For this review, take the finished solid that the model builds, in its own axes (mm). A direction names the side the tool comes from. Give positions to 0.01 mm unless a question says otherwise; leave off trailing zeros. Write each loop counter-clockwise with the first axis right and the second up, starting at its lowest first coordinate (ties: lowest second). Pieces come first, ordered by that corner, then holes.
from build123d import *

# Parameters (mm, degrees)
F0_W      = 38.1
F0_H      = 38.1
F1_DEPTH  = 0.79375
F2_W      = 38.1
F2_H      = 38.1
F2_W_2    = 34.8996
F2_H_2    = 34.8996
F3_DEPTH  = 5.08
F4_W      = 1.27
F4_H      = 10.9915577808
F4_H_2    = 10.7192572
F5_DEPTH  = 4.445
F7_W      = 1.27
F7_H      = 6.305353716
F9_DEPTH  = 4.445
F8_W      = 1.27
F8_H      = 7.127109261
F8_H_2    = 15.866300866
F8_W_2    = 9.8573208662
F8_H_3    = 1.27
F10_DEPTH = 4.445
F11_W     = 8.128
F11_H     = 1.27
F12_DEPTH = 4.445


# Not quite as in the source:
# - a feature names something its author has since deleted; it is built from what else it names


with BuildPart() as f1:
    # F0 (on Top) → F1 (new body)
    with BuildSketch(Plane.XY):
        with Locations((0.9067468345, -3.6591270581)):
            Rectangle(F0_W, F0_H)
    extrude(amount=F1_DEPTH)

    # F2 (on face) → F3 (join)
    with BuildSketch(Plane.XY.offset(0.79375)):
        with Locations((0.9067468345, -3.6591270581)):
            Rectangle(F2_W, F2_H)
        with Locations((0.9067468345, -3.6591270581)):
            Rectangle(F2_W_2, F2_H_2, mode=Mode.SUBTRACT)
    extrude(amount=F3_DEPTH)

    # F4 (on face) → F5 (join)
    with BuildSketch(Plane.XY.offset(0.79375)):
        with Locations((-10.8280531655, -15.6836010049)):
            Rectangle(F4_W, F4_H)
        Polygon((-11.4630531655, -5.1078221145), (-10.1930531655, -5.1078221145), (-10.1930531655, 1.8014254137), (-10.1930531655, 3.0714254137), (-10.1930531655, 8.7106729419), (-11.4630531655, 8.7106729419), align=None)
        Polygon((-10.1930531655, 3.0714254137), (-10.1930531655, 1.8014254137), (-3.8430531655, 1.8014254137), (-3.8430531655, 3.0714254137), (-5.1130531655, 3.0714254137), align=None)
        with Locations((-4.4780531655, 8.4310540137)):
            Rectangle(F4_W, F4_H_2)
    extrude(amount=F5_DEPTH)

    # F7 (on face) → F9 (join)
    with BuildSketch(Plane.XY.offset(0.79375)):
        Polygon((2.6555440854, -10.197567645), (-10.6428060681, -10.197567645), (-10.6428060681, -11.467567645), (-3.9936309913, -11.467567645), (-3.9936309913, -16.0289270581), (-2.7236309913, -16.0289270581), (-2.7236309913, -11.467567645), (2.6555440854, -11.467567645), align=None)
        with Locations((2.6458618774, -19.700244503)):
            Rectangle(F7_W, F7_H)
    extrude(amount=F9_DEPTH)

    # F8 (on face) → F10 (join)
    with BuildSketch(Plane.XY.offset(0.79375)):
        with Locations((1.5678320881, -7.4372278345)):
            Rectangle(F8_W, F8_H)
        Polygon((12.3628337599, 8.1913313339), (-4.464668509, 8.1913313339), (-4.464668509, 6.9213313339), (7.2828320881, 6.9213313339), (8.5528320881, 6.9213313339), (12.3628337599, 6.9213313339), align=None)
        with Locations((7.9178320881, -1.0118190991)):
            Rectangle(F8_W, F8_H_2)
        with Locations((13.370096651, -14.6599695321)):
            Rectangle(F8_W_2, F8_H_3)
    extrude(amount=F10_DEPTH)

    # F11 (on face) → F12 (join)
    with BuildSketch(Plane.XY.offset(0.79375)):
        with Locations((11.246104741, -1.0928286647)):
            Rectangle(F11_W, F11_H)
    extrude(amount=F12_DEPTH)


solid = f1.part
(1) We need section B-B (y = -17.5). Write out the cut boundary in (x, z), and give its area (3 significant figures).
(2) For L1, parallel to Y at x = -9.5, z = 3.6; L2, parallel to X at y = -15.5, z = 4.6; L3, parallel to Y at x = 16, z = 3.7, list the stretches that pass through material, from the lowest coordinate up.
(3) Tool access review of faces 1 (the flat face through (-1, -22, 5.874)), 2 (the flat face through (0.933, -7, 3)): name each direction out of +Z, -Z, +X, -X, +Y, -Y from which nothing blocks a thin tool from reaching the whole face with its end or side.
(4) We need section C-C (z = 2.15). Count the separate pieces of the cut face and the enclosed holes in it, and give its area (3 significant figures).
(5) We need section A-A (x = 6.5). Write out the cut boundary in (y, z).
(6) Clearance check with flat-ended pins moving along their axes: pin 1 Ø1.5 at (x, y) = (-14.5, 11) entering from +Z; pin 2 Ø15.5 at (x, y) = (-2.5, -10.5) entering from +Z; pin 3 Ø0.6 at (x, z) = (-3.5, 4) entering from -Y. State where each tip first meets the part, or that it passes through.
(7) The part is to be moulded in two halves that separate along Y. For faces 3 (the flat face through (3, -19, 5.239)), 4 (the flat face through (1, -3, 0)), say which applies: +Y half, -Y half, draft (parallel to the pull), parting line (faces both ways), or undercut.
(8) We need section D-D (x = -15). Write out the cut boundary in (y, z).
The answers:
1. outline: (-18.14, 0) - (19.96, 0) - (19.96, 5.87) - (18.36, 5.87) - (18.36, 0.79) - (3.28, 0.79) - (3.28, 5.24) - (2.01, 5.24) - (2.01, 0.79) - (-10.19, 0.79) - (-10.19, 5.24) - (-11.46, 5.24) - (-11.46, 0.79) - (-16.54, 0.79) - (-16.54, 5.87) - (-18.14, 5.87) - close
1. area: 57.8 mm2
2. L1: y = -22.71 to -21.11, -11.47 to -10.2, 1.8 to 3.07, 13.79 to 15.39
2. L2: x = -18.14 to -16.54, -11.46 to -10.19, -3.99 to -2.72, 18.36 to 19.96
2. L3: y = -22.71 to -21.11, -15.29 to -14.02, 13.79 to 15.39
3. face 1: +Z, +X, -X, +Y, -Y
3. face 2: +Z
4. separate pieces: 2
4. enclosed holes: 1
4. area: 385 mm2
5. outline: (-22.71, 0) - (15.39, 0) - (15.39, 5.87) - (13.79, 5.87) - (13.79, 0.79) - (8.19, 0.79) - (8.19, 5.24) - (6.92, 5.24) - (6.92, 0.79) - (-21.11, 0.79) - (-21.11, 5.87) - (-22.71, 5.87) - close
6. pin 1: stops at z = 0.79
6. pin 2: stops at z = 5.24
6. pin 3: stops at y = -22.71
7. face 3: undercut
7. face 4: draft
8. outline: (-22.71, 0) - (15.39, 0) - (15.39, 5.87) - (13.79, 5.87) - (13.79, 0.79) - (-21.11, 0.79) - (-21.11, 5.87) - (-22.71, 5.87) - close
